```python
from build123d import *

# Parameters (mm, degrees)
F0_W     = 15
F0_H     = 2
F1_DEPTH = 6.9
F3_DEPTH = 3.45


with BuildPart() as f1:
    # F0 (on Top) → F1 (new body)
    with BuildSketch(Plane.XY):
        with Locations((0, 7.25)):
            Rectangle(F0_W, F0_H)
    extrude(amount=F1_DEPTH)

    # F2 (on Top) → F3 (cut)
    with BuildSketch(Plane.XY):
        Polygon((-4.76314, 8.25), (-5.91784, 6.25), (-3.608439, 6.25), (-2.453739, 8.25), align=None)
        Polygon((3.608439, 6.25), (5.91784, 6.25), (4.76314, 8.25), (2.453739, 8.25), align=None)
    extrude(amount=F3_DEPTH, mode=Mode.SUBTRACT)


solid = f1.part
```
The listing builds one solid part. Answer for the finished solid, in the listing's coordinates (mm). A direction names the side the tool comes from. Give positions to 0.01 mm unless a question says otherwise; leave off trailing zeros. Write each loop counter-clockwise with the first axis right and the second up, starting at its lowest first coordinate (ties: lowest second). Pieces come first, ordered by that corner, then holes. Notation, with made-up numbers: (60, 0) -> (76, 0) arc R21 cw to (76, 5) -> close; hole circle Ø11 at (77, 26). An arc over 180 degrees is marked (long way). Use one line per item in the form item = value.
1) Section C-C on y = 7.1 is taken. Write down the section's boundary in (x, z).
Result:
outline = (-7.5, 0) -> (-5.43, 0) -> (-5.43, 3.45) -> (-3.12, 3.45) -> (-3.12, 0) -> (3.12, 0) -> (3.12, 3.45) -> (5.43, 3.45) -> (5.43, 0) -> (7.5, 0) -> (7.5, 6.9) -> (-7.5, 6.9) -> close
2) This flat-tipped pin is pushed along its axis until it touches: P1, Ø1, axis at x = -4.5, y = 7, coming from the -Z side. Where does it stop, or does it pass through?
Result:
P1 = 3.45
3) For a pull along X with two mould halves and no side action, classify faces 5 (the flat face through (-7.5, 7, 3)), 6 (the flat face through (-3.039, 7.236, 1.701)), 7 (the flat face through (-6, 7, 0)) as +X half, -X half, draft (parallel to the pull), parting line (faces both ways), or undercut.
Result:
face_5 = -X half
face_6 = undercut
face_7 = draft
4) Section A-A on z = 2.5 is taken. Write down the section's boundary in (x, y), plus the area to 3 significant figures.
Result:
outline = (-7.5, 6.25) -> (-5.92, 6.25) -> (-4.76, 8.25) -> (-7.5, 8.25) -> close; (-3.61, 6.25) -> (3.61, 6.25) -> (2.45, 8.25) -> (-2.45, 8.25) -> close; (4.76, 8.25) -> (5.92, 6.25) -> (7.5, 6.25) -> (7.5, 8.25) -> close
area = 20.8 mm²
5) A tool of negligible diameter and unlimited length cuts with its end or side. For faces 1 (the flat face through (5.349, 7.236, 1.701)), 2 (the flat face through (-4, 7, 3.45)), 3 (the flat face through (0, 6.25, 3)), 4 (the flat face through (3, 7.3, 1.7)), from which of +Z, -Z, +X, -X, +Y, -Y can it reach the whole face along a straight path? Write none if from no direction.
Result:
face_1 = -Z, -Y
face_2 = -Z
face_3 = +Z, -Z, +X, -X, -Y
face_4 = -Z, +Y
6) Straight lines are drawn through the part: probe 1 along X at (y, z) = (7.55, 1.5); probe 2 along Z at (x, y) = (-4.75, 7.1); probe 3 along X at (y, z) = (8, 3). For each, find the intervals that lie inside material, in ascending order.
Result:
probe_1 = -7.5 to -5.17, -2.86 to 2.86, 5.17 to 7.5
probe_2 = 3.45 to 6.9
probe_3 = -7.5 to -4.91, -2.6 to 2.6, 4.91 to 7.5
7) Section B-B on x = 4 is taken. Write down the section's boundary in (y, z), plus the area to 3 significant figures.
Result:
outline = (6.25, 3.45) -> (8.25, 3.45) -> (8.25, 6.9) -> (6.25, 6.9) -> close
area = 6.90 mm²
